from build123d import *

# Parameters (mm, degrees)
F0_R     = 148.5
F0_R_2   = 6.5786
F0_R_3   = 8.3312
F1_DEPTH = 20
F2_R     = 146.5
F2_R_2   = 142
F3_DEPTH = 5


# Not quite as in the source:
# - a feature names something its author has since deleted; it is built from what else it names


with BuildPart() as f1:
    # F0 (on Top) → F1 (new body)
    with BuildSketch(Plane.XY):
        Circle(F0_R)
        with Locations((-25, 43.3012701892)):
            Circle(F0_R_2, mode=Mode.SUBTRACT)
        Circle(F0_R_3, mode=Mode.SUBTRACT)
        with Locations((25, 43.3012701892)):
            Circle(F0_R_2, mode=Mode.SUBTRACT)
    extrude(amount=F1_DEPTH)

    # F2 (on face) → F3 (cut)
    with BuildSketch(Plane.XY):
        Circle(F2_R)
        Circle(F2_R_2, mode=Mode.SUBTRACT)
    extrude(amount=F3_DEPTH, mode=Mode.SUBTRACT)


solid = f1.part
Part model, mm, in its own coordinate system. A direction names the side the tool comes from. Coordinates: 2 decimals unless noted, no trailing zeros. Order: outer loops, then holes, each group sorted by start corner. A loop starts at its lowest first (then second) coordinate and runs counter-clockwise, first axis right, second up. Notation, with made-up numbers: M 16.5,55 L 27.5,55 A23 cw 27.5,77 Z; hole C 37.25,-35 d10. An arc over 180 degrees is marked long. Use a Markdown table: item, result.
(1) Cut at A-A on x = 0. Write the cut outline in (y, z), then the cut area to 3 significant figures.
A:
| item | result |
|---|---|
| outline | M -148.5,0 L -146.5,0 L -146.5,5 L -142,5 L -142,0 L -8.33,0 L -8.33,20 L -148.5,20 Z; M 8.33,0 L 142,0 L 142,5 L 146.5,5 L 146.5,0 L 148.5,0 L 148.5,20 L 8.33,20 Z |
| area | 5,560 mm^2 |
(2) Cut at B-B on y = -95.5. Write the cut outline in (x, z).
A:
| item | result |
|---|---|
| outline | M -113.72,0 L -111.09,0 L -111.09,5 L -105.09,5 L -105.09,0 L 105.09,0 L 105.09,5 L 111.09,5 L 111.09,0 L 113.72,0 L 113.72,20 L -113.72,20 Z |
(3) Pull direction Y, two halves, no side cores. Call faces 1 (the cylindrical face through (-19.332, 147.236, 9.86)), 2 (the flat face through (30, 2, 0)), 3 (the cylindrical face through (-25.856, 49.824, 9.86)): released by +Y, released by -Y, zero draft, split by the parting line, or undercut.
A:
| item | result |
|---|---|
| face 1 | split by the parting line |
| face 2 | zero draft |
| face 3 | undercut |
(4) Probe L1, parallel to Y at x = 0, z = 2.8; L2, parallel to Z at x = 46, y = -135; L3, parallel to Y at x = 85.5, z = 4.5. List the from-to ranges inside material, lowest first.
A:
| item | result |
|---|---|
| L1 | y = -148.5 to -146.5, -142 to -8.33, 8.33 to 142, 146.5 to 148.5 |
| L2 | z = 5 to 20 |
| L3 | y = -121.42 to -118.96, -113.37 to 113.37, 118.96 to 121.42 |
(5) Flat gauge pins, fed straight in: pin 1 (6 mm diameter, centred on x = 34.5, z = 10.5, fed in from -Y); pin 2 (5 mm diameter, centred on x = -18, z = 14.5, fed in from -Y); pin 3 (2 mm diameter, centred on y = -83, z = 17.5, fed in from -X); pin 4 (13.5 mm diameter, centred on x = 0, y = 0, fed in from -Z). Where does each tip first touch, or does it go through?
A:
| item | result |
|---|---|
| pin 1 | stops at y = -145.12 |
| pin 2 | stops at y = -147.69 |
| pin 3 | stops at x = -123.81 |
| pin 4 | passes through |
(6) Tool access for faces 4 (the flat face through (31, 2, 20)), 5 (the cylindrical face through (-30.783, -138.623, 2.465)): list every direction of +Z, -Z, +X, -X, +Y, -Y with a clear straight run to the whole face (end or side of a thin tool).
A:
| item | result |
|---|---|
| face 4 | +Z, +X, -X, +Y, -Y |
| face 5 | -Z |
(7) Cut at D-D on z = 16.75. Write the cut outline in (x, y), then the cut area to 3 significant figures.
A:
| item | result |
|---|---|
| outline | C 0,0 d297; hole C -25,43.3 d13.16; hole C 0,0 d16.66; hole C 25,43.3 d13.16 |
| area | 68,800 mm^2 |
(8) Cut at C-C on x = 86. Write the cut outline in (y, z).
A:
| item | result |
|---|---|
| outline | M -121.06,0 L -118.6,0 L -118.6,5 L -113,5 L -113,0 L 113,0 L 113,5 L 118.6,5 L 118.6,0 L 121.06,0 L 121.06,20 L -121.06,20 Z |
